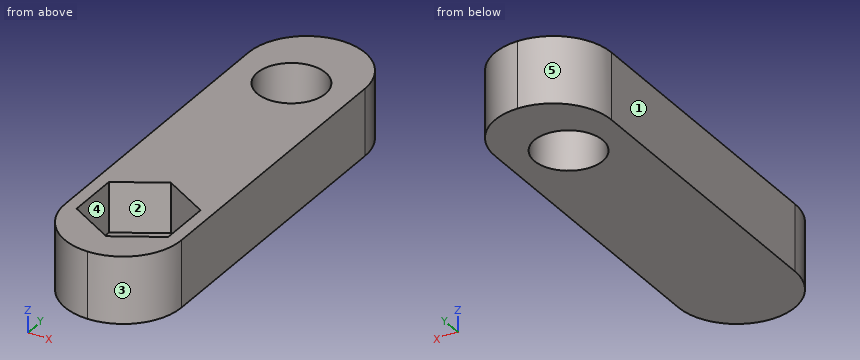
from build123d import *

# Parameters (mm, degrees)
F0_R     = 2.05
F1_DEPTH = 1
F2_DEPTH = 3
F3_R     = 3.49999


# Not quite as in the source:
# - a fillet or chamfer is up to 0.001 mm smaller than in the source, because OpenCascade refuses the exact size


with BuildPart() as f1:
    # F0 (on Top) → F1 (new body)
    with BuildSketch(Plane.XY):
        Polygon((-3.5, -20), (3.5, -20), (3.5, 5), (0, 5), (-3.5, 5), align=None)
        Polygon((0, -18.1754264805), (-2.75, -16.5877132403), (-2.75, -13.4122867597), (0, -11.8245735195), (2.75, -13.4122867597), (2.75, -16.5877132403), align=None, mode=Mode.SUBTRACT)
        Circle(F0_R, mode=Mode.SUBTRACT)
        Polygon((-2.75, -13.4122867597), (-2.75, -16.5877132403), (0, -18.1754264805), (2.75, -16.5877132403), (2.75, -13.4122867597), (0, -11.8245735195), align=None)
    extrude(amount=-F1_DEPTH)

    # F0 (on Top) → F2 (join)
    with BuildSketch(Plane.XY):
        Polygon((-3.5, -20), (3.5, -20), (3.5, 5), (0, 5), (-3.5, 5), align=None)
        Polygon((0, -18.1754264805), (-2.75, -16.5877132403), (-2.75, -13.4122867597), (0, -11.8245735195), (2.75, -13.4122867597), (2.75, -16.5877132403), align=None, mode=Mode.SUBTRACT)
        Circle(F0_R, mode=Mode.SUBTRACT)
    extrude(amount=F2_DEPTH)

    # F3 (radius 3.5 in the source; OpenCascade refuses exactly that, so slightly less here)
    f3_edges = [f1.edges().sort_by_distance(p)[0] for p in [
        (3.5, -20, 1),
        (-3.5, -20, 1),
        (3.5, 5, 1),
        (-3.5, 5, 1),
    ]]
    fillet(f3_edges, radius=F3_R)


solid = f1.part
The model under review builds one solid part; all positions refer to its coordinate system, in mm. Face numbers are marked on the shaded views. A direction names the side the tool comes from. Round coordinates to 2 decimals unless told otherwise and drop trailing zeros. Order: outer loops, then holes, each group sorted by start corner. A loop starts at its lowest first (then second) coordinate and runs counter-clockwise, first axis right, second up. Notation, with made-up numbers: (-16.5, 69) -> (41.5, 69) arc R24 ccw to (41.5, 91) -> close; hole circle Ø6 at (46.5, -2.75). An arc over 180 degrees is marked (long way). Use CSV: the item, a comma, the result in double quotes. Start each with the question number.
(1) Consider section C-C on x = -2.5. Write out the cut boundary in (y, z).
(2) Consider section A-A on z = 2.1. State how many separate pieces and enclosed holes the cut face has, and give its area (3 significant figures).
(3) Consider section B-B on x = -0.25. Write out the cut boundary in (y, z).
(4) Consider section D-D on x = 3.25. Write out the cut boundary in (y, z).
(5) Insertion check: pin 1 (1.6 mm diameter, centred on x = 0, y = -13.5, fed in from +Z); pin 2 (1 mm diameter, centred on x = 2, y = 0, fed in from +Z). Each pin has a flat end and moves straight along its axis. Give the tip position at first contact, or say it passes through.
(6) Tool access review of the marked faces 1 and 2: name each direction out of +Z, -Z, +X, -X, +Y, -Y from which nothing blocks a thin tool from reaching the whole face with its end or side.
(7) Wall thickness on probe 1 along X at (y, z) = (-16, 1); probe 2 along Y at (x, z) = (-0.5, 0.5); probe 3 along Z at (x, y) = (-0.25, -14.75): over which ranges is each line inside the solid? List them lowest first. Write a range as from..to.
(8) Mouldability with a two-part tool opening along X and no side actions: class the marked faces 3, 4 and 5 as pulls with the +X half, pulls with the -X half, needs draft (parallel to the pull), parting line crosses it, or undercut.
Responses:
1,outline,"(-18.95, -1) -> (3.95, -1) -> (3.95, 3) -> (-13.27, 3) -> (-13.27, 0) -> (-16.73, 0) -> (-16.73, 3) -> (-18.95, 3) -> close"
2,separate pieces,"1"
2,enclosed holes,"2"
2,area,"125 mm²"
3,outline,"(-19.99, -1) -> (-2.03, -1) -> (-2.03, 3) -> (-11.97, 3) -> (-11.97, 0) -> (-18.03, 0) -> (-18.03, 3) -> (-19.99, 3) -> close; (2.03, -1) -> (4.99, -1) -> (4.99, 3) -> (2.03, 3) -> close"
4,outline,"(-17.8, -1) -> (2.8, -1) -> (2.8, 3) -> (-17.8, 3) -> close"
5,pin 1,"z = 0"
5,pin 2,"z = 3"
6,face 1,"+Z, -Z, -X, +Y, -Y"
6,face 2,"+Z"
7,probe 1,"-3.5..-2.75, 2.75..3.5"
7,probe 2,"-19.96..-17.89, -12.11..-1.99, 1.99..4.96"
7,probe 3,"-1..0"
8,face 3,"pulls with the +X half"
8,face 4,"undercut"
8,face 5,"pulls with the -X half"
